from build123d import *

# Parameters (mm, degrees)
SKETCH_1_W          = 101
SKETCH_1_H          = 74
EXTRUDE_1_DEPTH     = 3
EXTRUDE_START       = 1.5
SKETCH_2_W          = 107
SKETCH_2_H          = 80
EXTRUDE_2_DEPTH     = 1.5
SKETCH_3_W          = 10.4
SKETCH_3_H          = 10.4
CUT_EXTRUDE_1_DEPTH = 5


with BuildPart() as part:
    # Эскиз1 → Бобышка-Вытянуть1 (new body)
    with BuildSketch(Plane.XY):
        with Locations((53.5, 40)):
            Rectangle(SKETCH_1_W, SKETCH_1_H)
    extrude(amount=EXTRUDE_1_DEPTH)

    # Эскиз2 → Бобышка-Вытянуть2 (add)
    with BuildSketch(Plane.XY.offset(EXTRUDE_START)):
        with Locations((53.5, 40)):
            Rectangle(SKETCH_2_W, SKETCH_2_H)
    extrude(amount=EXTRUDE_2_DEPTH)

    # Эскиз3 → Вырез-Вытянуть1 (cut)
    with BuildSketch(Plane.XY.offset(3)):
        with Locations((29.8, 68.15)):
            Rectangle(SKETCH_3_W, SKETCH_3_H)
        with Locations((45.533, 68.15)):
            Rectangle(SKETCH_3_W, SKETCH_3_H)
        with Locations((61.267, 68.15)):
            Rectangle(SKETCH_3_W, SKETCH_3_H)
        with Locations((77, 68.15)):
            Rectangle(SKETCH_3_W, SKETCH_3_H)
        with BuildLine():
            Line((25.5, 19.3), (82.2, 19.3))
            ThreePointArc((82.2, 19.3), (88.2, 13.3), (82.2, 7.3))
            Line((82.2, 7.3), (25.5, 7.3))
            ThreePointArc((25.5, 7.3), (19.5, 13.3), (25.5, 19.3))
        make_face()
    extrude(amount=-CUT_EXTRUDE_1_DEPTH, mode=Mode.SUBTRACT)


solid = part.part
Verification items for the finished model (mm, model axes). Give positions to 0.01 mm unless a question says otherwise; leave off trailing zeros. Order: outer loops, then holes, each group sorted by start corner. A loop starts at its lowest first (then second) coordinate and runs counter-clockwise, first axis right, second up. Notation, with made-up numbers: M 35,-31.75 L 78,-31.75 A6 cw 78,-22.75 Z; hole C 18.25,-28 d2. An arc over 180 degrees is marked long. Answer as a JSON object with one key per item and string values. Group by question number.
1) Cross-section at C-C (z = 0.95). Enter the section's corners in (x, y), then the cut area to 3 significant figures.
2) Cross-section at A-A (y = 13.3). Enter the section's corners in (x, z), then the cut area to 3 significant figures.
3) Scan lines: line 1 along X through (y, z) = (65, 2.55); line 2 along Y through (x, z) = (74, 2.25); line 3 along Y through (x, z) = (59, 0.9). Record each from-to range of solid material in increasing order. Write a range as [from, to].
4) Mould release check, pull along Y, two halves, no side actions. Record for faces 1 (the face through (53, 41, 3)), 2 (the face through (50.733, 68, 2)): released by +Y, released by -Y, zero draft, split by the parting line, or undercut.
5) Cross-section at D-D (y = 23.5). Enter the section's corners in (x, z), then the cut area to 3 significant figures.
6) Cross-section at B-B (x = 60). Enter the section's corners in (y, z), then the cut area to 3 significant figures.
Result sheet:
{
 "1": {"outline": "M 3,3 L 104,3 L 104,77 L 3,77 Z; hole M 24.6,62.95 L 35,62.95 L 35,73.35 L 24.6,73.35 Z; hole M 25.5,7.3 L 82.2,7.3 A6 ccw 82.2,19.3 L 25.5,19.3 A6 ccw Z; hole M 40.33,62.95 L 50.73,62.95 L 50.73,73.35 L 40.33,73.35 Z; hole M 56.07,62.95 L 66.47,62.95 L 66.47,73.35 L 56.07,73.35 Z; hole M 71.8,62.95 L 82.2,62.95 L 82.2,73.35 L 71.8,73.35 Z", "area": "6,250 mm2"},
 "2": {"outline": "M 0,1.5 L 3,1.5 L 3,0 L 19.5,0 L 19.5,3 L 0,3 Z; M 88.2,0 L 104,0 L 104,1.5 L 107,1.5 L 107,3 L 88.2,3 Z", "area": "106 mm2"},
 "3": {"line 1": "x = [0, 24.6], [35, 40.33], [50.73, 56.07], [66.47, 71.8], [82.2, 107]", "line 2": "y = [0, 7.3], [19.3, 62.95], [73.35, 80]", "line 3": "y = [3, 7.3], [19.3, 62.95], [73.35, 77]"},
 "4": {"face 1": "zero draft", "face 2": "undercut"},
 "5": {"outline": "M 0,1.5 L 3,1.5 L 3,0 L 104,0 L 104,1.5 L 107,1.5 L 107,3 L 0,3 Z", "area": "312 mm2"},
 "6": {"outline": "M 0,1.5 L 3,1.5 L 3,0 L 7.3,0 L 7.3,3 L 0,3 Z; M 19.3,0 L 62.95,0 L 62.95,3 L 19.3,3 Z; M 73.35,0 L 77,0 L 77,1.5 L 80,1.5 L 80,3 L 73.35,3 Z", "area": "164 mm2"}
}
